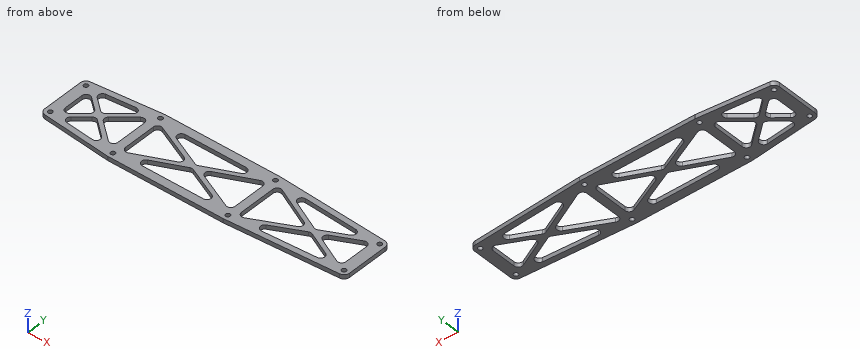
from build123d import *

# Parameters (mm, degrees)
SKETCH_1_W          = 232
SKETCH_1_H          = 56
SKETCH_1_R          = 1.6
EXTRUDE_1_DEPTH     = 3
SKETCH_2_R          = 1.6
CUT_EXTRUDE_1_DEPTH = 10
SKETCH_4_W          = 232
SKETCH_4_H          = 56
CUT_EXTRUDE_2_DEPTH = 5
CUT_EXTRUDE_3_DEPTH = 5
FILLET_1_R          = 3


with BuildPart() as part:
    # 草图1 → 凸台-拉伸1 (new body)
    with BuildSketch(Plane.XY):
        Rectangle(SKETCH_1_W, SKETCH_1_H)
        with Locations((-56.5, 20)):
            Circle(SKETCH_1_R, mode=Mode.SUBTRACT)
        with Locations((-56.5, -20)):
            Circle(SKETCH_1_R, mode=Mode.SUBTRACT)
        with Locations((26.5, -20)):
            Circle(SKETCH_1_R, mode=Mode.SUBTRACT)
        with Locations((26.5, 20)):
            Circle(SKETCH_1_R, mode=Mode.SUBTRACT)
    extrude(amount=EXTRUDE_1_DEPTH)

    # 草图2 → 切除-拉伸1 (cut)
    with BuildSketch(Plane.XY.offset(3)):
        with Locations((-106, 15)):
            Circle(SKETCH_2_R)
        with Locations((-106, -15)):
            Circle(SKETCH_2_R)
        with Locations(Location((106, -15, 0), (0, 0, 180))):
            Circle(SKETCH_2_R)
        with Locations(Location((106, 15, 0), (0, 0, 180))):
            Circle(SKETCH_2_R)
    extrude(amount=-CUT_EXTRUDE_1_DEPTH, mode=Mode.SUBTRACT)

    # 草图4 → 切除-拉伸2 (cut, symmetric)
    with BuildSketch(Plane.XY.offset(3)):
        Rectangle(SKETCH_4_W, SKETCH_4_H)
        with BuildLine():
            ThreePointArc((106.251076246, 18.992112313), (108.915845073, 17.73821977), (110, 15))
            Line((110, 15), (110, -15))
            ThreePointArc((110, -15), (108.915845073, -17.73821977), (106.251076246, -18.992112313))
            Line((106.251076246, -18.992112313), (26.751076246, -23.992112313))
            ThreePointArc((26.751076246, -23.992112313), (26.625600057, -23.998027592), (26.5, -24))
            Line((26.5, -24), (-56.5, -24))
            ThreePointArc((-56.5, -24), (-56.701252299, -23.994933981), (-56.901994824, -23.979748756))
            Line((-56.901994824, -23.979748756), (-106.401994824, -18.979748756))
            ThreePointArc((-106.401994824, -18.979748756), (-108.967151774, -17.682538043), (-110, -15))
            Line((-110, -15), (-110, 15))
            ThreePointArc((-110, 15), (-108.967151774, 17.682538043), (-106.401994824, 18.979748756))
            Line((-106.401994824, 18.979748756), (-56.901994824, 23.979748756))
            ThreePointArc((-56.901994824, 23.979748756), (-56.701252299, 23.994933981), (-56.5, 24))
            Line((-56.5, 24), (26.5, 24))
            ThreePointArc((26.5, 24), (26.625600057, 23.998027592), (26.751076246, 23.992112313))
            Line((26.751076246, 23.992112313), (106.251076246, 18.992112313))
        make_face(mode=Mode.SUBTRACT)
    extrude(amount=CUT_EXTRUDE_2_DEPTH, both=True, mode=Mode.SUBTRACT)

    # 草图6 → 切除-拉伸3 (cut, symmetric)
    with BuildSketch(Plane.XY.offset(3)):
        Polygon((-63.143230899, 19.328966576), (-99.922202515, 15.613918938), (-83.735209235, 1.962237858), align=None)
        Polygon((-60.5, 17.633721737), (-81.408555774, 0), (-60.5, -17.633721737), align=None)
        Polygon((-63.143230899, -19.328966576), (-83.735209235, -1.962237858), (-99.922202515, -15.613918938), align=None)
        Polygon((-86.061862696, 0), (-102, 13.441802546), (-102, -13.441802546), align=None)
        Polygon((-18.617329048, 0), (-54.5, 16.351596889), (-54.5, -16.351596889), align=None)
        Polygon((20.882670952, 18), (-50.882670952, 18), (-15, 1.648403111), align=None)
        Polygon((24.5, 16.351596889), (-11.382670952, 0), (24.5, -16.351596889), align=None)
        Polygon((20.882670952, -18), (-15, -1.648403111), (-50.882670952, -18), align=None)
        Polygon((67.431494542, 0), (30.5, 18.078353971), (30.5, -18.078353971), align=None)
        Polygon((98.97671451, 15.441716069), (34.414687191, 19.502220931), (70.843216532, 1.670073702), align=None)
        Polygon((102, 13.581498626), (74.254938522, 0), (102, -13.581498626), align=None)
        Polygon((98.97671451, -15.441716069), (70.843216532, -1.670073702), (34.414687191, -19.502220931), align=None)
    extrude(amount=CUT_EXTRUDE_3_DEPTH, both=True, mode=Mode.SUBTRACT)

    # 圆角1
    fillet_1_edges = [part.edges().sort_by_distance(p)[0] for p in [
        (-11.382670952, 0, 1.5),
        (24.5, 16.351596889, 1.5),
        (24.5, -16.351596889, 1.5),
        (-15, 1.648403111, 1.5),
        (-50.882670952, 18, 1.5),
        (20.882670952, 18, 1.5),
        (-50.882670952, -18, 1.5),
        (-15, -1.648403111, 1.5),
        (20.882670952, -18, 1.5),
        (30.5, -18.078353971, 1.5),
        (30.5, 18.078353971, 1.5),
        (67.431494542, 0, 1.5),
        (-83.735209235, -1.962237858, 1.5),
        (-63.143230899, -19.328966576, 1.5),
        (-99.922202515, -15.613918938, 1.5),
        (-60.5, 17.633721737, 1.5),
        (-60.5, -17.633721737, 1.5),
        (-81.408555774, 0, 1.5),
        (-86.061862696, 0, 1.5),
        (-102, -13.441802546, 1.5),
        (-102, 13.441802546, 1.5),
        (-54.5, -16.351596889, 1.5),
        (-54.5, 16.351596889, 1.5),
        (-18.617329048, 0, 1.5),
        (34.414687191, -19.502220931, 1.5),
        (70.843216532, -1.670073702, 1.5),
        (98.97671451, -15.441716069, 1.5),
        (70.843216532, 1.670073702, 1.5),
        (34.414687191, 19.502220931, 1.5),
        (98.97671451, 15.441716069, 1.5),
        (74.254938522, 0, 1.5),
        (102, 13.581498626, 1.5),
        (102, -13.581498626, 1.5),
        (-99.922202515, 15.613918938, 1.5),
        (-63.143230899, 19.328966576, 1.5),
        (-83.735209235, 1.962237858, 1.5),
    ]]
    fillet(fillet_1_edges, radius=FILLET_1_R)


solid = part.part
For this review, take the finished solid that the model builds, in its own axes (mm). Give positions to 0.01 mm unless a question says otherwise; leave off trailing zeros. Loops run counter-clockwise (first coordinate to the right, second up) from the corner with the lowest first, then second, coordinate; pieces in that order, holes last. Notation, with made-up numbers: M -25,23.25 L -12,23.25 A30 ccw -12,52.25 Z; hole C 72,56.5 d11. An arc over 180 degrees is marked long. Answer as a JSON object with one key per item and string values. Group by question number.
Q1. Insertion check: P1, Ø2.5, axis at x = -56.5, y = -20, coming from the +Z side. The pin has a flat end and moves straight along its axis. Give the tip position at first contact, or say it passes through.
Q2. Add section B-B on x = 95. Give the boundary of the cut face in (y, z), and give its area (3 significant figures).
Q3. For probe 1 along Y at (x, z) = (26.5, 1.4); probe 2 along Y at (x, z) = (106, 0.6); probe 3 along Y at (x, z) = (47, 1.7), list the stretches that pass through material, from the lowest coordinate up. Write a range as [from, to].
Q4. Add section C-C on z = 0.5. Give the number of separate pieces and of enclosed holes in the cut face, and give its area (3 significant figures).
Q5. Add section A-A on x = 4.5. Give the boundary of the cut face in (y, z).
Q6. Add section D-D on x = 38. Give the boundary of the cut face in (y, z).
Checked values:
{
 "1": {"P1": "through"},
 "2": {"outline": "M -19.7,0 L -10.15,0 L -10.15,3 L -19.7,3 Z; M 10.15,0 L 19.7,0 L 19.7,3 L 10.15,3 Z", "area": "57.3 mm²"},
 "3": {"probe 1": "[-24, -21.6], [-18.4, 18.4], [21.6, 24]", "probe 2": "[-19.01, -16.6], [-13.4, 13.4], [16.6, 19.01]", "probe 3": "[-22.72, -17.5], [-13.62, -10], [10, 13.62], [17.5, 22.72]"},
 "4": {"separate pieces": "1", "enclosed holes": "20", "area": "4,630 mm²"},
 "5": {"outline": "M -24,0 L -18,0 L -18,3 L -24,3 Z; M -10.53,0 L -7.24,0 L -7.24,3 L -10.53,3 Z; M 7.24,0 L 10.53,0 L 10.53,3 L 7.24,3 Z; M 18,0 L 24,0 L 24,3 L 18,3 Z"},
 "6": {"outline": "M -23.28,0 L -14.41,0 L -14.41,3 L -23.28,3 Z; M 14.41,0 L 23.28,0 L 23.28,3 L 14.41,3 Z"}
}
